Input: part model. Units: mm. Frame: model coordinates. A direction names the side the tool comes from. Coordinates: 2 decimals unless noted, no trailing zeros. One line per question, with ' | ' between items. Start each with the question number.
```python
from build123d import *

# Parameters (mm, degrees)
SKETCH1_W                      = 118
SKETCH1_H                      = 8
EXTRUDE1_DEPTH                 = 200
F_4_5_4_5_DIAMETER_HOLE1_D     = 4.5
F_4_5_4_5_DIAMETER_HOLE1_DEPTH = 20
F_4_5_4_5_DIAMETER_HOLE1_TIP   = 1.351936393
F_4_5_4_5_DIAMETER_HOLE2_D     = 4.5
F_4_5_4_5_DIAMETER_HOLE2_DEPTH = 20
F_4_5_4_5_DIAMETER_HOLE2_TIP   = 1.351936393


with BuildPart() as part:
    # Sketch1 → Extrude1 (new body)
    with BuildSketch(Plane(origin=(0, 0, 0), x_dir=(1, 0, 0), z_dir=(0, 1, 0))):
        with Locations((59, 4)):
            Rectangle(SKETCH1_W, SKETCH1_H)
    extrude(amount=EXTRUDE1_DEPTH)

    # Ø4.5 (4.5) Diameter Hole1
    with Locations(Plane(origin=(23, 200, -4), x_dir=(0, 0, 1), z_dir=(0, 1, 0))):
        with Locations((0, 0), (0, 80)):
            Hole(F_4_5_4_5_DIAMETER_HOLE1_D / 2, depth=F_4_5_4_5_DIAMETER_HOLE1_DEPTH)
            with Locations((0, 0, -(F_4_5_4_5_DIAMETER_HOLE1_DEPTH + F_4_5_4_5_DIAMETER_HOLE1_TIP / 2))):  # 118° drill point
                Cone(0, F_4_5_4_5_DIAMETER_HOLE1_D / 2, F_4_5_4_5_DIAMETER_HOLE1_TIP, mode=Mode.SUBTRACT)

    # Ø4.5 (4.5) Diameter Hole2
    with Locations(Plane(origin=(23, 0, -4), x_dir=(0, 0, -1), z_dir=(0, -1, 0))):
        with Locations((0, 0), (0, 80)):
            Hole(F_4_5_4_5_DIAMETER_HOLE2_D / 2, depth=F_4_5_4_5_DIAMETER_HOLE2_DEPTH)
            with Locations((0, 0, -(F_4_5_4_5_DIAMETER_HOLE2_DEPTH + F_4_5_4_5_DIAMETER_HOLE2_TIP / 2))):  # 118° drill point
                Cone(0, F_4_5_4_5_DIAMETER_HOLE2_D / 2, F_4_5_4_5_DIAMETER_HOLE2_TIP, mode=Mode.SUBTRACT)


solid = part.part
```
(1) Reachability of faces 4 (the face through (20.804, 189.86, -3.512)), 5 (the face through (58, 200, -4)), 6 (the face through (100.804, 10.14, -4.488)) from +Z, -Z, +X, -X, +Y, -Y: full face, straight path, thin tool, end or side. Return the list, or none.
(2) Draft query along X for faces 1 (the face through (58, 99, 0)), 2 (the face through (0, 99, -4)), 3 (the face through (20.804, 10.14, -4.488)). Return one class per face: +X half, -X half, draft (parallel to the pull), parting line (faces both ways), or undercut.
(3) Pin query (flat end, axial travel): pin 1 (2.5 mm diameter, centred on x = 23, z = -4, fed in from -Y); pin 2 (4 mm diameter, centred on x = 103, z = -4, fed in from -Y). Return the tip coordinate at first contact, or that it passes through.
(4) Material intervals for line 1 along X through (y, z) = (193, -4); line 2 along Z through (x, y) = (103, 7.5); line 3 along X through (y, z) = (182.5, -2.25), sorted ascending. Write a range as from..to.
Worked answers:
1) face 4: +Y | face 5: +Z, -Z, +X, -X, +Y | face 6: -Y
2) face 1: draft | face 2: -X half | face 3: undercut
3) pin 1: stops at y = 20.6 | pin 2: stops at y = 20.15
4) line 1: x = 0..20.75, 25.25..100.75, 105.25..118 | line 2: z = -8..-6.25, -1.75..0 | line 3: x = 0..21.59, 24.41..101.59, 104.41..118
